from build123d import *

# Parameters (mm, degrees)
SKETCH1_R                = 29.0703
BOSS_EXTRUDE2_DEPTH      = 4.7625
FILLET1_R                = 3.175
SKETCH2_W                = 14.732
SKETCH2_H                = 10.414
CUT_EXTRUDE2_DEPTH       = 12.7
CIRPATTERN1_COUNT        = 7
SKETCH4_R                = 1.143
CUT_EXTRUDE4_DEPTH       = 9.525
CIRPATTERN2_COUNT        = 7
SKETCH6_R                = 2.286
CUT_EXTRUDE7_DEPTH       = 42.376236281
SKETCH7_R                = 4.445
CUT_EXTRUDE8_DEPTH       = 2.54
BOSS_EXTRUDE4_REACH      = 48.843
FILLET2_R                = 0.127
CIRPATTERN5_COUNT        = 7
FILLET2_OF_CIRPATTERN5_R = 0.127
SKETCH5_R                = 6
CUT_EXTRUDE9_DEPTH       = 5.08
SKETCH11_R               = 6
SKETCH11_R_2             = 5
BOSS_EXTRUDE5_DEPTH      = 1.27


with BuildPart() as part:
    # Sketch1 → Boss-Extrude2 (new body)
    with BuildSketch(Plane.XY):
        Circle(SKETCH1_R)
    extrude(amount=-BOSS_EXTRUDE2_DEPTH)

    # Fillet1
    fillet1_edges = [part.edges().sort_by_distance(p)[0] for p in [
        (-29.0703, 0, -4.7625),
    ]]
    fillet(fillet1_edges, radius=FILLET1_R)

    # Sketch2 → Cut-Extrude2 (cut)
    with BuildSketch(Plane.XY):
        with Locations((0, 25.1333)):
            Rectangle(SKETCH2_W, SKETCH2_H)
    cut_extrude2 = extrude(amount=-CUT_EXTRUDE2_DEPTH, mode=Mode.SUBTRACT)

    # CirPattern1: Cut-Extrude2 ×7 about axis
    cirpattern1_axis = Axis((0, 0, 0), (0, 0, 1))
    for i in range(1, CIRPATTERN1_COUNT):
        add(cut_extrude2.rotate(cirpattern1_axis, i * 360 / CIRPATTERN1_COUNT), mode=Mode.SUBTRACT)

    # Sketch4 → Cut-Extrude4 (cut, symmetric)
    with BuildSketch(Plane(origin=(0, 0, 0), x_dir=(0, 0, -1), z_dir=(1, 0, 0))):
        with Locations((0, 25.7683)):
            Circle(SKETCH4_R)
    cut_extrude4 = extrude(amount=CUT_EXTRUDE4_DEPTH, both=True, mode=Mode.SUBTRACT)

    # CirPattern2: Cut-Extrude4 ×7 about axis
    cirpattern2_axis = Axis((0, 0, 0), (0, 0, 1))
    for i in range(1, CIRPATTERN2_COUNT):
        add(cut_extrude4.rotate(cirpattern2_axis, i * 360 / CIRPATTERN2_COUNT), mode=Mode.SUBTRACT)

    # Sketch6 → Cut-Extrude7 (cut, through all)
    with BuildSketch(Plane(origin=(0, 0, -4.7625), x_dir=(-1, 0, 0), z_dir=(0, 0, -1))):
        with Locations((12.7, 0)):
            Circle(SKETCH6_R)
        with Locations((0, -12.7)):
            Circle(SKETCH6_R)
        with Locations((-12.7, 0)):
            Circle(SKETCH6_R)
        with Locations((0, 12.7)):
            Circle(SKETCH6_R)
    extrude(amount=-CUT_EXTRUDE7_DEPTH, mode=Mode.SUBTRACT)

    # Sketch7 → Cut-Extrude8 (cut)
    with BuildSketch(Plane(origin=(0, 0, -4.7625), x_dir=(-1, 0, 0), z_dir=(0, 0, -1))):
        with Locations((12.7, 0)):
            Circle(SKETCH7_R)
        with Locations((0, -12.7)):
            Circle(SKETCH7_R)
        with Locations((-12.7, 0)):
            Circle(SKETCH7_R)
        with Locations((0, 12.7)):
            Circle(SKETCH7_R)
    extrude(amount=-CUT_EXTRUDE8_DEPTH, mode=Mode.SUBTRACT)

    # Sketch10 → Boss-Extrude4 (add, up to next)
    with BuildSketch(Plane.ZY.offset(-7.366), mode=Mode.PRIVATE) as boss_extrude4_sk1:
        with BuildLine():
            Line((-4.7625, 19.9263), (0, 19.9263))
            Line((0, 19.9263), (0, 20.0533))
            ThreePointArc((0, 20.0533), (-2.7025038, 20.73265722), (-4.7625, 22.609214887))
            Line((-4.7625, 22.609214887), (-4.7625, 19.9263))
        make_face()
    boss_extrude4_tool1 = extrude(boss_extrude4_sk1.sketch, amount=BOSS_EXTRUDE4_REACH, mode=Mode.PRIVATE) - part.part
    boss_extrude4 = boss_extrude4_tool1.solids().sort_by_distance((7.366, 20.664807, -3.452063))[0]
    add(boss_extrude4)

    # Fillet2
    fillet2_edges = [part.edges().sort_by_distance(p)[0] for p in [
        (0, 22.609214887, -4.7625),
    ]]
    fillet(fillet2_edges, radius=FILLET2_R)

    # CirPattern5: Boss-Extrude4 ×7 about axis
    cirpattern5_axis = Axis((0, 0, 0), (0, 0, 1))
    for i in range(1, CIRPATTERN5_COUNT):
        add(boss_extrude4.rotate(cirpattern5_axis, i * 360 / CIRPATTERN5_COUNT))

    # Fillet2 of CirPattern5
    fillet2_of_cirpattern5_edges = [part.edges().sort_by_distance(p)[0] for p in [
        (-17.676595993, 14.09661491, -4.7625),
        (-22.042354666, -5.031023613, -4.7625),
        (-9.809770694, -20.370198741, -4.7625),
        (9.809770694, -20.370198741, -4.7625),
        (22.042354666, -5.031023613, -4.7625),
        (17.676595993, 14.09661491, -4.7625),
    ]]
    fillet(fillet2_of_cirpattern5_edges, radius=FILLET2_OF_CIRPATTERN5_R)

    # Sketch5 → Cut-Extrude9 (cut)
    with BuildSketch(Plane.XY):
        Circle(SKETCH5_R)
    extrude(amount=-CUT_EXTRUDE9_DEPTH, mode=Mode.SUBTRACT)

    # Sketch11 → Boss-Extrude5 (add)
    with BuildSketch(Plane.XY):
        Circle(SKETCH11_R)
        Circle(SKETCH11_R_2, mode=Mode.SUBTRACT)
    extrude(amount=-BOSS_EXTRUDE5_DEPTH)


solid = part.part
Geometry check sheet. Reference: the model listing, model coordinates, mm. A direction names the side the tool comes from. Round coordinates to 2 decimals unless told otherwise and drop trailing zeros. One line per question, with ' | ' between items. Start each with the question number.
1. Scan lines: line 1 (X direction, y = 23.5, z = -3.1); line 2 (Y direction, x = 0, z = -0.35); line 3 (X direction, y = 9, z = -3.7). Record each from-to range of solid material in increasing order. Write a range as [from, to].
2. Cross-section at A-A on z = -3.75. State how many separate pieces and enclosed holes the cut face has, then the cut area to 3 significant figures.
3. Tool access check on faces 5 (the face through (25.068, 1.834, -2.348)), 6 (the face through (-14.196, 20.742, -2.348)), 7 (the face through (-23.381, 9.224, -2.348)), 8 (the face through (0.96, 8.36, -3.51)), 9 (the face through (-22.78, -18.06, -0.78)). Record the directions out of +Z, -Z, +X, -X, +Y, -Y that give a thin tool (end or side, any length) a straight path to the whole face; none if there is none.
4. Draft check along Y on faces 1 (the face through (-18.792, -19.523, -1.143)), 2 (the face through (22.679, -18.186, -0.783)), 3 (the face through (-13, 26, -1)), 4 (the face through (-3.574, -26.852, -1.143)). Enter one of: released by +Y, released by -Y, zero draft, split by the parting line, or undercut.
5. Depth check by flat-ended pin: pin 1 (0.9 mm diameter, centred on y = 26, z = -0.5, fed in from +X); pin 2 (1.5 mm diameter, centred on y = 6, z = -4, fed in from -X); pin 3 (7 mm diameter, centred on x = 1.5, y = -13, fed in from -Z); pin 4 (2.5 mm diameter, centred on x = -2, y = 11, fed in from -Z). Enter the tip coordinate at first touch or a pass-through.
Taken from the geometry:
1) line 1: [-16.45, -7.37], [7.37, 16.45] | line 2: [-29.07, -14.99], [-10.41, -5], [5, 10.41], [14.99, 20.06] | line 3: [-26.79, -23.1], [-20.21, -2.46], [2.46, 20.21], [23.1, 26.79]
2) separate pieces: 1 | enclosed holes: 5 | area: 1,480 mm²
3) face 5: +Z | face 6: +Z, -X | face 7: +Z, +Y | face 8: -Z | face 9: +Z, -Z, -X, -Y
4) face 1: undercut | face 2: released by -Y | face 3: released by +Y | face 4: undercut
5) pin 1: x = 13.87 | pin 2: x = -27.99 | pin 3: z = -4.76 | pin 4: z = -2.22
